Here's how the part is built. I have some questions about the finished solid (model axes, mm). Face numbers are marked on the shaded views. A direction names the side the tool comes from. Give positions to 0.01 mm unless a question says otherwise; leave off trailing zeros. Write each loop counter-clockwise with the first axis right and the second up, starting at its lowest first coordinate (ties: lowest second). Pieces come first, ordered by that corner, then holes. Notation, with made-up numbers: (20.25, 17) -> (25.25, 17) arc R9 ccw to (25.25, 27) -> close; hole circle Ø3 at (72, -35.75). An arc over 180 degrees is marked (long way). Use CSV: the item, a comma, the result in double quotes. Start each with the question number.
(1) I need wall thicknesses on L1, parallel to Z at x = -5, y = 28 (3 decimals); L2, parallel to Z at x = -26.5, y = -1; L3, parallel to X at y = 32, z = -11 (3 decimals). Which ranges of each line are inside material? Lowest first, please. Write a range as [from, to].
(2) Suppose I cut it at D-D on y = 20. List the corners of the cut face in (x, z) for me, plus the area to 3 significant figures.
(3) If we mould it in two halves opening along Y, with no side actions, what happens to the marked faces 1, 2, 3 and 4? For each: pulls with the +Y half, pulls with the -Y half, needs draft (parallel to the pull), parting line crosses it, or undercut.
(4) Suppose I cut it at C-C on x = -18. List the corners of the cut face in (y, z) for me, plus the area to 3 significant figures.
(5) Which directions (+Z, -Z, +X, -X, +Y, -Y) give clear straight access to the entire face, cutting with the end or side of a thin tool? Please do the marked faces 5, 6 and 7.
(6) For pin 1 Ø4 at (x, z) = (-27, 9) entering from -Y; pin 2 Ø3 at (y, z) = (-16.5, 7) entering from -X; pin 3 Ø3.5 at (x, z) = (-5, 11) entering from +Y; pin 4 Ø3.5 at (x, z) = (-29, -11) entering from -Y, each with a flat end and sliding along its axis, tell me the tip position at first contact or that it passes through.
(7) Suppose I cut it at A-A on y = -20. List the corners of the cut face in (x, z) for me.
(8) Suppose I cut it at B-B on z = -6. List the corners of the cut face in (x, y) for me, plus the area to 3 significant figures.
from build123d import *

# Parameters (mm, degrees)
SKETCH1_W           = 28.5
SKETCH1_H           = 46.5
SKETCH1_R           = 1.5
SKETCH1_R_2         = 10.875
BOSS_EXTRUDE1_DEPTH = 1
SKETCH2_W           = 34
SKETCH2_H           = 28.5
BOSS_EXTRUDE2_DEPTH = 6.5
CUT_EXTRUDE1_REACH  = 66.04
SKETCH4_R           = 4.175
SKETCH15_W          = 34
SKETCH15_H          = 28.5
SKETCH15_R          = 2.15
BOSS_EXTRUDE8_DEPTH = 5
CHAMFER1_SIZE       = 6.5
BOSS_EXTRUDE9_DEPTH = 2
SKETCH5_R           = 2.5
BOSS_EXTRUDE4_DEPTH = 5
CUT_EXTRUDE4_START  = -5
SKETCH7_R           = 1.6
CUT_EXTRUDE4_DEPTH  = 5
SKETCH10_R          = 2.075
BOSS_EXTRUDE6_DEPTH = 12.25
CUT_EXTRUDE7_START  = -10
SKETCH18_R          = 2.075
CUT_EXTRUDE7_DEPTH  = 10
SKETCH19_R          = 4
CUT_EXTRUDE8_DEPTH  = 3


with BuildPart() as part:
    # Sketch1 → Boss-Extrude1 (new, symmetric)
    with BuildSketch(Plane(origin=(0, 0, 0), x_dir=(0, 0, -1), z_dir=(1, 0, 0))):
        Rectangle(SKETCH1_W, SKETCH1_H)
        with Locations((-11, 20)):
            Circle(SKETCH1_R, mode=Mode.SUBTRACT)
        with Locations(Location((11, 20, 0), (0, 0, 180))):
            Circle(SKETCH1_R, mode=Mode.SUBTRACT)
        with Locations((11, -20)):
            Circle(SKETCH1_R, mode=Mode.SUBTRACT)
        with Locations(Location((-11, -20, 0), (0, 0, 180))):
            Circle(SKETCH1_R, mode=Mode.SUBTRACT)
        with Locations((0, 12)):
            Circle(SKETCH1_R_2, mode=Mode.SUBTRACT)
    extrude(amount=BOSS_EXTRUDE1_DEPTH, both=True)

    # Sketch2 → Boss-Extrude2 (add)
    with BuildSketch(Plane(origin=(0, 23.25, 0), x_dir=(1, 0, 0), z_dir=(0, 1, 0))):
        with Locations((-16, 0)):
            Rectangle(SKETCH2_W, SKETCH2_H)
    extrude(amount=BOSS_EXTRUDE2_DEPTH)

    # Sketch4 → Cut-Extrude1 (cut, up to next)
    with BuildSketch(Plane(origin=(0, 29.75, 0), x_dir=(1, 0, 0), z_dir=(0, 1, 0)), mode=Mode.PRIVATE) as cut_extrude1_sk1:
        with Locations(Location((-16.75, 0, 0), (0, 0, 270))):
            Circle(SKETCH4_R)
    cut_extrude1_tool1 = extrude(cut_extrude1_sk1.sketch, amount=-CUT_EXTRUDE1_REACH, mode=Mode.PRIVATE) & part.part
    add(cut_extrude1_tool1.solids().sort_by_distance((-16.75, 29.75, 0))[0], mode=Mode.SUBTRACT)

    # Sketch15 → Boss-Extrude8 (add)
    with BuildSketch(Plane.XZ.offset(23.25)):
        with Locations((-16, 0)):
            Rectangle(SKETCH15_W, SKETCH15_H)
        with Locations(Location((-12.75, 0, 0), (0, 0, 270))):
            Circle(SKETCH15_R, mode=Mode.SUBTRACT)
    extrude(amount=BOSS_EXTRUDE8_DEPTH)

    # Chamfer1
    chamfer1_edges = [part.edges().sort_by_distance(p)[0] for p in [
        (1, 29.75, 0),
    ]]
    chamfer(chamfer1_edges, length=CHAMFER1_SIZE)

    # Sketch17 → Boss-Extrude9 (add)
    with BuildSketch(Plane.XY.offset(14.25)):
        Polygon((-33, 29.75), (-33, -28.25), (1, -28.25), (1, 23.25), (-5.5, 29.75), align=None)
    boss_extrude9 = extrude(amount=BOSS_EXTRUDE9_DEPTH)

    # Mirror3: Boss-Extrude9 across plane
    add(boss_extrude9.mirror(Plane.XY))

    # Sketch5 → Boss-Extrude4 (add)
    with BuildSketch(Plane(origin=(12.125, 12.125, 0), x_dir=(0, 0, -1), z_dir=(0.7071067811865487, 0.7071067811865464, 0))):
        with Locations(Location((0, 20.329319959, 0), (0, 0, 90))):
            Circle(SKETCH5_R)
    extrude(amount=BOSS_EXTRUDE4_DEPTH)

    # Sketch7 → Cut-Extrude4 (cut)
    with BuildSketch(Plane(origin=(15.660533906, 15.660533906, 0), x_dir=(0, 0, -1), z_dir=(0.7071067811865487, 0.7071067811865464, 0)).offset(CUT_EXTRUDE4_START)):
        with Locations(Location((0, 20.329319959, 0), (0, 0, 90))):
            Circle(SKETCH7_R)
    extrude(amount=CUT_EXTRUDE4_DEPTH, mode=Mode.SUBTRACT)

    # Sketch10 → Boss-Extrude6 (add)
    with BuildSketch(Plane(origin=(0, 23.25, 0), x_dir=(1, 0, 0), z_dir=(0, 1, 0))):
        with BuildLine():
            Line((-33, -16.25), (-33, 16.25))
            Line((-33, 16.25), (-6.654581397, 16.25))
            ThreePointArc((-6.654581397, 16.25), (-2.942270796, 14.712310601), (-1.404581397, 11))
            ThreePointArc((-1.404581397, 11), (-3.679011202, 7.656046722), (-7.624732517, 8.542803601))
            ThreePointArc((-7.624732517, 8.542803601), (-29.25, 0), (-7.624732517, -8.542803601))
            ThreePointArc((-7.624732517, -8.542803601), (-3.679011202, -7.656046722), (-1.404581397, -11))
            ThreePointArc((-1.404581397, -11), (-2.942270796, -14.712310601), (-6.654581397, -16.25))
            Line((-6.654581397, -16.25), (-33, -16.25))
        make_face()
        with Locations(Location((-29, 11, 0), (0, 0, 90))):
            Circle(SKETCH10_R, mode=Mode.SUBTRACT)
        with Locations(Location((-29, -11, 0), (0, 0, 90))):
            Circle(SKETCH10_R, mode=Mode.SUBTRACT)
        with Locations(Location((-5, 11, 0), (0, 0, 103.943434861))):
            Circle(SKETCH10_R, mode=Mode.SUBTRACT)
        with Locations(Location((-5, -11, 0), (0, 0, 103.943434861))):
            Circle(SKETCH10_R, mode=Mode.SUBTRACT)
    extrude(amount=BOSS_EXTRUDE6_DEPTH)

    # Sketch18 → Cut-Extrude7 (cut)
    with BuildSketch(Plane(origin=(0, 35.5, 0), x_dir=(1, 0, 0), z_dir=(0, 1, 0)).offset(CUT_EXTRUDE7_START)):
        with Locations(Location((-5, -11, 0), (0, 0, 270))):
            Circle(SKETCH18_R)
        with Locations(Location((-5, 11, 0), (0, 0, 270))):
            Circle(SKETCH18_R)
    extrude(amount=CUT_EXTRUDE7_DEPTH, mode=Mode.SUBTRACT)

    # Sketch19 → Cut-Extrude8 (cut)
    with BuildSketch(Plane.XZ.offset(28.25)):
        with Locations((-5.75, 17.85)):
            Circle(SKETCH19_R)
        with Locations((-5.75, -17.85)):
            Circle(SKETCH19_R)
        with Locations(Location((-27.35, 8.14, 0), (0, 0, 270))):
            Circle(SKETCH19_R)
        with Locations(Location((-27.35, -8.14, 0), (0, 0, 270))):
            Circle(SKETCH19_R)
    extrude(amount=-CUT_EXTRUDE8_DEPTH, mode=Mode.SUBTRACT)


solid = part.part
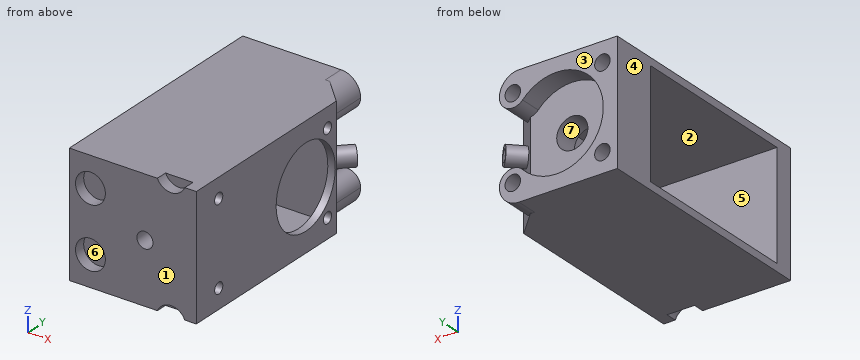
Geometry says:
1,L1,"[-16.25, -13.075], [-8.925, 8.925], [13.075, 16.25]"
1,L2,"[-16.25, -14.25], [14.25, 16.25]"
1,L3,"[-33, -31.075], [-26.925, -22.687], [-10.813, -7.075], [-2.925, -1.405]"
2,outline,"(-33, -16.25) -> (1, -16.25) -> (1, -12.5) -> (-1, -12.5) -> (-1, -14.25) -> (-33, -14.25) -> close; (-33, 14.25) -> (-1, 14.25) -> (-1, 12.5) -> (1, 12.5) -> (1, 16.25) -> (-33, 16.25) -> close; (-1, -9.5) -> (1, -9.5) -> (1, -7.37) -> (-1, -7.37) -> close; (-1, 7.37) -> (1, 7.37) -> (1, 9.5) -> (-1, 9.5) -> close"
2,area,"152 mm²"
3,face 1,"pulls with the -Y half"
3,face 2,"undercut"
3,face 3,"pulls with the +Y half"
3,face 4,"needs draft"
4,outline,"(-28.25, -16.25) -> (35.5, -16.25) -> (35.5, -12.44) -> (29.75, -12.44) -> (29.75, -3.98) -> (23.25, -3.98) -> (23.25, -14.25) -> (-23.25, -14.25) -> (-23.25, 14.25) -> (23.25, 14.25) -> (23.25, 3.98) -> (29.75, 3.98) -> (29.75, 12.44) -> (35.5, 12.44) -> (35.5, 16.25) -> (-28.25, 16.25) -> close"
4,area,"552 mm²"
5,face 5,"-X"
5,face 6,"-Y"
5,face 7,"+Y"
6,pin 1,"y = -25.25"
6,pin 2,"x = -1"
6,pin 3,"y = 25.5"
6,pin 4,"y = -28.25"
7,outline,"(-33, -16.25) -> (1, -16.25) -> (1, -12.5) -> (-1, -12.5) -> (-1, -14.25) -> (-33, -14.25) -> close; (-33, 14.25) -> (-1, 14.25) -> (-1, 12.5) -> (1, 12.5) -> (1, 16.25) -> (-33, 16.25) -> close; (-1, -9.5) -> (1, -9.5) -> (1, 9.5) -> (-1, 9.5) -> close"
8,outline,"(-33, -28.25) -> (-30.73, -28.25) -> (-30.73, -25.25) -> (-23.97, -25.25) -> (-23.97, -28.25) -> (1, -28.25) -> (1, 2.93) -> (-1, 2.93) -> (-1, -23.25) -> (-33, -23.25) -> close; (-33, 23.25) -> (-1, 23.25) -> (-1, 21.07) -> (1, 21.07) -> (1, 23.25) -> (-5.5, 29.75) -> (-27.72, 29.75) -> (-27.72, 35.5) -> (-33, 35.5) -> close"
8,area,"437 mm²"
